The model under review builds one solid part; all positions refer to its coordinate system, in mm. Face numbers are marked on the shaded views. A direction names the side the tool comes from. Coordinates: 2 decimals unless noted, no trailing zeros. Write each loop counter-clockwise with the first axis right and the second up, starting at its lowest first coordinate (ties: lowest second). Pieces come first, ordered by that corner, then holes. Notation, with made-up numbers: (2.5, -40) -> (37.5, -40) arc R8 ccw to (37.5, -34) -> close; hole circle Ø9 at (-6, 74.5). An arc over 180 degrees is marked (long way). Put each result on its own line as item: value. Start each with the question number.
from build123d import *

# Parameters (mm, degrees)
SKETCH_2_OUTSIDE_W  = 43.8
SKETCH_2_OUTSIDE_H  = 43.8
CUT_EXTRUDE_1_DEPTH = 47.16275555


with BuildPart() as part:
    # Эскиз1 → Повернуть1 (revolve)
    with BuildSketch(Plane.XY, mode=Mode.PRIVATE) as revolve_1_sk:
        with BuildLine():
            Line((0, 2), (0, 4.4))
            Line((0, 4.4), (1.6, 6))
            Line((1.6, 6), (10.75, 6))
            Line((10.75, 6), (11.853553391, 4.896446609))
            ThreePointArc((11.853553391, 4.896446609), (12.015765065, 4.788060234), (12.207106781, 4.75))
            Line((12.207106781, 4.75), (15, 4.75))
            ThreePointArc((15, 4.75), (15.707106781, 5.042893219), (16, 5.75))
            Line((16, 5.75), (16, 11))
            Line((16, 11), (18.309401077, 15))
            Line((18.309401077, 15), (38.690598923, 15))
            Line((38.690598923, 15), (41, 11))
            Line((41, 11), (41, 9))
            Line((41, 9), (39, 7))
            Line((39, 7), (26.5, 7))
            Line((26.5, 7), (25.146446609, 8.353553391))
            ThreePointArc((25.146446609, 8.353553391), (24.984234935, 8.461939766), (24.792893219, 8.5))
            Line((24.792893219, 8.5), (22, 8.5))
            ThreePointArc((22, 8.5), (21.292893219, 8.207106781), (21, 7.5))
            Line((21, 7.5), (21, 4))
            Line((21, 4), (19, 2))
            Line((19, 2), (0, 2))
        make_face()
    revolve(revolve_1_sk.sketch.rotate(Axis((0, 0, 0), (1, 0, 0)), 90), axis=Axis((0, 0, 0), (1, 0, 0)))

    # Эскиз2 outside → Вырез-Вытянуть1 (cut, through all)
    with BuildSketch(Plane(origin=(41, 0, 0), x_dir=(0, 0, -1), z_dir=(1, 0, 0))):
        Rectangle(SKETCH_2_OUTSIDE_W, SKETCH_2_OUTSIDE_H)
        Polygon((0, 15.588457268), (-13.5, 7.794228634), (-13.5, -7.794228634), (0, -15.588457268), (13.5, -7.794228634), (13.5, 7.794228634), align=None, mode=Mode.SUBTRACT)
    extrude(amount=-CUT_EXTRUDE_1_DEPTH, mode=Mode.SUBTRACT)


solid = part.part
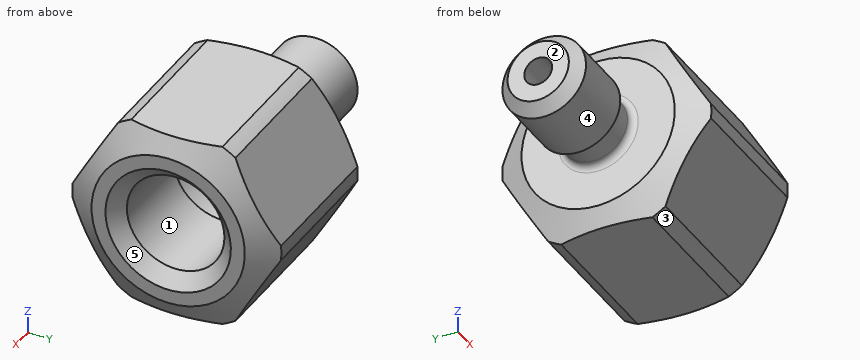
1. Consider section B-B on x = 27. State the section outline as (y, z) points, then the cut area to 3 significant figures.
2. Wall thickness on line 1 (Y direction, x = 23.4, z = 0); line 2 (Y direction, x = 10.5, z = 0); line 3 (X direction, y = -0.25, z = -9.25): over which ranges is each line inside the solid? List them lowest first. Write a range as from..to.
3. The part is to be moulded in two halves that separate along Z. For the marked faces 3, 4 and 5, say which applies: released by +Z, released by -Z, zero draft, split by the parting line, or undercut.
4. Insertion check: P1, Ø6, axis at y = 8, z = -5.5, coming from the -X side; P2, Ø1.5, axis at x = 25, y = 7.5, coming from the -Z side; P3, Ø12.5, axis at y = 0, z = 0, coming from the +X side. Each pin has a flat end and moves straight along its axis. Give the tip position at first contact, or say it passes through.
5. Consider section A-A on x = 20. State the section outline as (y, z) points.
6. Tool access review of the marked faces 1 and 2: name each direction out of +Z, -Z, +X, -X, +Y, -Y from which nothing blocks a thin tool from reaching the whole face with its end or side.
7. Consider section C-C on x = 10. State the section outline as (y, z) points.
Output values:
1. outline: (-14.96, -1.09) -> (-8.42, -12.41) arc R15 ccw to (-6.54, -13.5) -> (6.54, -13.5) arc R15 ccw to (8.42, -12.41) -> (14.96, -1.09) arc R15 ccw to (14.96, 1.09) -> (8.42, 12.41) arc R15 ccw to (6.54, 13.5) -> (-6.54, 13.5) arc R15 ccw to (-8.42, 12.41) -> (-14.96, 1.09) arc R15 ccw to start; hole circle Ø14 at (0, 0)
1. area: 474 mm^2
2. line 1: y = -15..-8.5, 8.5..15
2. line 2: y = -6..-2, 2..6
2. line 3: x = 16..41
3. face 3: released by -Z
3. face 4: split by the parting line
3. face 5: undercut
4. P1: stops at x = 16
4. P2: stops at z = -13.4
4. P3: stops at x = 21
5. outline: (-14.96, -1.09) -> (-8.42, -12.41) arc R15 ccw to (-6.54, -13.5) -> (6.54, -13.5) arc R15 ccw to (8.42, -12.41) -> (14.96, -1.09) arc R15 ccw to (14.96, 1.09) -> (8.42, 12.41) arc R15 ccw to (6.54, 13.5) -> (-6.54, 13.5) arc R15 ccw to (-8.42, 12.41) -> (-14.96, 1.09) arc R15 ccw to start; hole circle Ø6 at (0, 0)
6. face 1: +X
6. face 2: +Z, -Z, -X, +Y, -Y
7. outline: circle Ø12 at (0, 0); hole circle Ø4 at (0, 0)
